Geometry check sheet. Reference: the model listing, model coordinates, mm. Face numbers are marked on the shaded views. A direction names the side the tool comes from. Round coordinates to 2 decimals unless told otherwise and drop trailing zeros. Order: outer loops, then holes, each group sorted by start corner. A loop starts at its lowest first (then second) coordinate and runs counter-clockwise, first axis right, second up. Notation, with made-up numbers: (-24, 65) -> (4, 65) arc R22 ccw to (4, 71) -> close; hole circle Ø4 at (-33, 43). An arc over 180 degrees is marked (long way). Answer as a JSON object with one key per item and string values. Group by question number.
from build123d import *

# Parameters (mm, degrees)
ESQUISSE1_W             = 74
ESQUISSE1_H             = 74
BOSS_EXTRU_1_DEPTH      = 32
BOSS_EXTRU_1_TAPER      = 5
ESQUISSE2_W             = 19.942710043
ESQUISSE2_H             = 22
ESQUISSE2_W_2           = 15.933949428
ENL_V_MAT_EXTRU_1_DEPTH = 29
ESQUISSE3_R             = 2.5
ENL_V_MAT_EXTRU_2_DEPTH = 10
ESQUISSE5_W             = 32
ESQUISSE5_H             = 15
BOSS_EXTRU_2_DEPTH      = 2


with BuildPart() as part:
    # Esquisse1 → Boss.-Extru.1 (new body)
    with BuildSketch(Plane.XY):
        with Locations((-135.106350006, 30.682970669)):
            Rectangle(ESQUISSE1_W, ESQUISSE1_H)
    extrude(amount=BOSS_EXTRU_1_DEPTH, taper=BOSS_EXTRU_1_TAPER)

    # Esquisse2 → Enlèv. mat.-Extru.1 (cut)
    with BuildSketch(Plane.XY.offset(32)):
        with Locations((-174.077705028, 30.682970669)):
            Rectangle(ESQUISSE2_W, ESQUISSE2_H)
        with Locations((-98.139375292, 30.682970669)):
            Rectangle(ESQUISSE2_W_2, ESQUISSE2_H)
    extrude(amount=-ENL_V_MAT_EXTRU_1_DEPTH, mode=Mode.SUBTRACT)

    # Esquisse3 → Enlèv. mat.-Extru.2 (cut)
    with BuildSketch(Plane.XY.offset(3)):
        with Locations((-167.606350006, 30.682970669)):
            Circle(ESQUISSE3_R)
        with Locations((-102.606350006, 30.682970669)):
            Circle(ESQUISSE3_R)
    extrude(amount=-ENL_V_MAT_EXTRU_2_DEPTH, mode=Mode.SUBTRACT)

    # Esquisse5 → Boss.-Extru.2 (add)
    with BuildSketch(Plane(origin=(0, 67.168842465, 5.876512258), x_dir=(1, 0, 0), z_dir=(0, 0.9961946980917457, 0.08715574274765837))):
        with Locations((-135.106350006, -1.60104042)):
            Rectangle(ESQUISSE5_W, ESQUISSE5_H)
    extrude(amount=BOSS_EXTRU_2_DEPTH)


solid = part.part
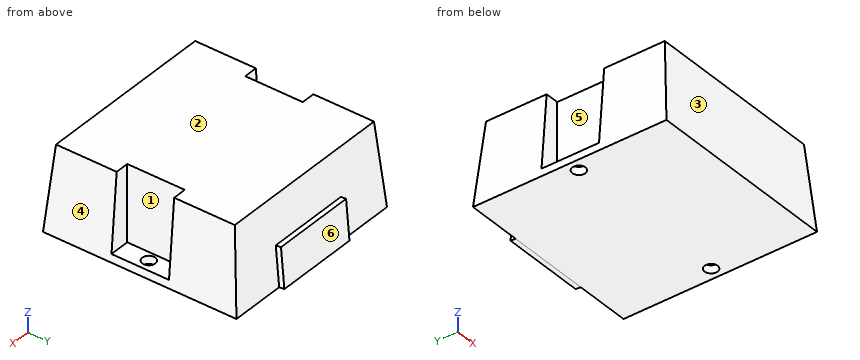
Item 1: Mould release check, pull along Y, two halves, no side actions. Record for the marked faces 3, 4, 5 and 6: pulls with the +Y half, pulls with the -Y half, needs draft (parallel to the pull), parting line crosses it, or undercut.
Item 2: Set-up check for the marked faces 1 and 2: record each of +Z, -Z, +X, -X, +Y, -Y from which the full face is reachable in a straight line by a thin tool's end or side.
Item 3: Sectioned sample at B-B, the plane x = -122.5. Enter the section's corners in (y, z).
Item 4: Sectioned sample at D-D, the plane z = 24.5. Enter the section's corners in (x, y), then the cut area to 3 significant figures.
Item 5: Depth check by flat-ended pin: pin 1 Ø1.5 at (y, z) = (58.5, 5) entering from +X; pin 2 Ø3.5 at (y, z) = (68.5, 4.5) entering from -X; pin 3 Ø6 at (x, z) = (-104, 19) entering from +Y; pin 4 Ø1.5 at (x, y) = (-141, 23) entering from -Z. Enter the tip coordinate at first touch or a pass-through.
Item 6: Sectioned sample at C-C, the plane x = -103. Enter the section's corners in (y, z).
Item 7: Thickness scan on L1, parallel to X at y = 31, z = 7; L2, parallel to Z at x = -169, y = 39.5; L3, parallel to Y at x = -116, z = 27. Record the ranges inside material, lowest first.
Item 8: Sectioned sample at A-A, the plane y = 38. Enter the section's corners in (x, z).
Result:
{
 "1": {"face 3": "pulls with the -Y half", "face 4": "needs draft", "face 5": "undercut", "face 6": "pulls with the +Y half"},
 "2": {"face 1": "+Z, +X", "face 2": "+Z, +X, -X, +Y, -Y"},
 "3": {"outline": "(-6.32, 0) -> (67.68, 0) -> (69.68, 0.17) -> (68.37, 15.12) -> (66.38, 14.94) -> (64.88, 32) -> (-3.52, 32) -> close"},
 "4": {"outline": "(-169.96, -4.17) -> (-100.25, -4.17) -> (-100.25, 19.68) -> (-106.11, 19.68) -> (-106.11, 41.68) -> (-100.25, 41.68) -> (-100.25, 65.54) -> (-169.96, 65.54) -> (-169.96, 41.68) -> (-164.11, 41.68) -> (-164.11, 19.68) -> (-169.96, 19.68) -> close", "area": "4,600 mm2"},
 "5": {"pin 1": "stops at x = -98.48", "pin 2": "stops at x = -171.83", "pin 3": "stops at y = 66.28", "pin 4": "stops at z = 0"},
 "6": {"outline": "(-6.32, 0) -> (28.21, 0) -> (28.21, 3) -> (19.68, 3) -> (19.68, 32) -> (-3.52, 32) -> close; (33.15, 0) -> (67.68, 0) -> (64.88, 32) -> (41.68, 32) -> (41.68, 3) -> (33.15, 3) -> close"},
 "7": {"L1": "x = -164.11 to -106.11", "L2": "z = 0 to 3", "L3": "y = -3.95 to 65.32"},
 "8": {"outline": "(-172.11, 0) -> (-98.11, 0) -> (-98.37, 3) -> (-106.11, 3) -> (-106.11, 32) -> (-164.11, 32) -> (-164.11, 3) -> (-171.84, 3) -> close"}
}
